from build123d import *

# Parameters (mm, degrees)
F1_DEPTH    = 6
F2_W        = 8.5644074716
F2_H        = 2.9347334579
F3_DEPTH    = 6
F5_DEPTH    = 25
F6_T1_DEPTH = 24.4869357348
F6_T3_DEPTH = 24.4827319302
F7_R        = 3
F8_R        = 1


# Not quite as in the source:
# - a fillet or chamfer that OpenCascade refuses, or shapes differently, is made with other operations: its cross-section is extruded or revolved along the edge and cut away or added


with BuildPart() as f1:
    # F0 (on Top) → F1 (new body)
    with BuildSketch(Plane.XY):
        Polygon((-4.42252215, 28.2665032521), (16.57747785, 28.2665032521), (16.57747785, -12.2334967479), (-4.42252215, -12.2334967479), (-4.42252215, -11.2334967479), (-5.42252215, -11.2334967479), (-5.42252215, -13.2334967479), (-5.42252215, -15.2334967479), (-4.42252215, -15.2334967479), (16.57747785, -15.2334967479), (19.57747785, -15.2334967479), (19.57747785, -13.2334967479), (19.57747785, 27.2665032521), (19.57747785, 31.2665032521), (16.57747785, 31.2665032521), (-4.42252215, 31.2665032521), (-5.42252215, 31.2665032521), (-5.42252215, 27.2665032521), (-4.42252215, 27.2665032521), align=None)
    extrude(amount=F1_DEPTH)

    # F2 (on face) → F3 (join)
    with BuildSketch(Plane.YZ.offset(19.57747785)):
        with Locations((7.0165032521, 3)):
            Rectangle(F2_W, F2_H)
    extrude(amount=F3_DEPTH)

    # F4 (on face) → F5 (cut)
    with BuildSketch(Plane.XY.offset(4.4673667289)):
        with BuildLine():
            Line((25.57747785, 8.833928965), (22.57747785, 9.2672181241))
            ThreePointArc((22.57747785, 9.2672181241), (20.32747785, 7.0172181241), (22.57747785, 4.7672181241))
            Line((22.57747785, 4.7672181241), (25.57747785, 5.2005072832))
            Line((25.57747785, 5.2005072832), (25.57747785, 8.833928965))
        make_face()
    extrude(amount=-F5_DEPTH, mode=Mode.SUBTRACT)

    # F6: fillet of radius 5 on 2 edges, made by hand

    # F6_s2 → F6_t1 (cut)
    with BuildSketch(Plane.XY.offset(-9.2434678674)):
        with BuildLine():
            ThreePointArc((21.2670373946, 2.7342995163), (23.7500837932, 3.3944284833), (25.57747785, 5.2005072832))
            Line((25.57747785, 5.2005072832), (25.57747785, 2.7342995163))
            Line((25.57747785, 2.7342995163), (21.2670373946, 2.7342995163))
        make_face()
    extrude(amount=F6_T1_DEPTH, mode=Mode.SUBTRACT)

    # F6_s4 → F6_t3 (cut)
    with BuildSketch(Plane.XY.offset(-9.2413659651)):
        with BuildLine():
            ThreePointArc((21.2678781556, 11.2987069879), (23.7502046967, 10.6389898062), (25.57747785, 8.833928965))
            Line((25.57747785, 8.833928965), (25.57747785, 11.2987069879))
            Line((25.57747785, 11.2987069879), (21.2678781556, 11.2987069879))
        make_face()
    extrude(amount=F6_T3_DEPTH, mode=Mode.SUBTRACT)

    # F7
    f7_edges = [f1.edges().sort_by_distance(p)[0] for p in [
        (19.577478, -15.233497, 3),
        (19.577478, 31.266503, 3),
    ]]
    fillet(f7_edges, radius=F7_R)

    # F8
    f8_edges = [f1.edges().sort_by_distance(p)[0] for p in [
        (-5.422522, -15.233497, 3),
        (-5.422522, 31.266503, 3),
        (23.750084, 3.394428, 4.467367),
        (23.750084, 3.394428, 1.532633),
        (23.750205, 10.63899, 1.532633),
        (23.750205, 10.63899, 4.467367),
        (20.422678, 11.298707, 1.532633),
        (20.422258, 2.7343, 1.532633),
        (20.422258, 2.7343, 4.467367),
        (20.422678, 11.298707, 4.467367),
    ]]
    fillet(f8_edges, radius=F8_R)


solid = f1.part
Input: part model. Units: mm. Frame: model coordinates. A direction names the side the tool comes from. Give positions to 0.01 mm unless a question says otherwise; leave off trailing zeros. Order: outer loops, then holes, each group sorted by start corner. A loop starts at its lowest first (then second) coordinate and runs counter-clockwise, first axis right, second up.
Q1. Section B-B on z = 1.05. Output: boundary loops of the cut face in (x, y), and give its area (3 significant figures).
Checked values:
outline: (-5.42, -14.23) arc R1 ccw to (-4.42, -15.23) - (16.58, -15.23) arc R3 ccw to (19.58, -12.23) - (19.58, 28.27) arc R3 ccw to (16.58, 31.27) - (-4.42, 31.27) arc R1 ccw to (-5.42, 30.27) - (-5.42, 27.27) - (-4.42, 27.27) - (-4.42, 28.27) - (16.58, 28.27) - (16.58, -12.23) - (-4.42, -12.23) - (-4.42, -11.23) - (-5.42, -11.23) - close
area: 269 mm2
Q2. Set-up query: faces 4 (the cylindrical face through (20.43, 11, 4.18)), 5 (the flat face through (20, 7, 1.533)), 6 (the flat face through (6, 28.267, 3)), 7 (the flat face through (-5, 27.267, 3)). Return all of +Z, -Z, +X, -X, +Y, -Y with unobstructed straight access to the full face (end or side cutting, diameter ignored); none if empty.
Checked values:
face 4: +Z, +X, +Y
face 5: -Z, +X, +Y, -Y
face 6: +Z, -Z
face 7: +Z, -Z, -X
Q3. Section C-C on y = 15. Output: boundary loops of the cut face in (x, z).
Checked values:
outline: (16.58, 0) - (19.58, 0) - (19.58, 6) - (16.58, 6) - close
Q4. Section A-A on x = 1. Output: boundary loops of the cut face in (y, z).
Checked values:
outline: (-15.23, 0) - (-12.23, 0) - (-12.23, 6) - (-15.23, 6) - close; (28.27, 0) - (31.27, 0) - (31.27, 6) - (28.27, 6) - close
Q5. Contact query for flat-ended pins moving along their axis: pin 1 Ø0.5 at (x, z) = (-5, 4.5) entering from +Y; pin 2 Ø0.8 at (x, z) = (-5, 4) entering from -Y; pin 3 Ø1.1 at (y, z) = (28, 4) entering from +X. Output: stop coordinate, or through.
Checked values:
pin 1: stops at y = 31.21
pin 2: stops at y = -15.22
pin 3: stops at x = 19.58
Q6. Ray query, probe 1 along Y at (x, z) = (3.5, 0.95); probe 2 along X at (y, z) = (27.5, 2.55); probe 3 along X at (y, z) = (-7, 2.9). Return the intervals inside material, ascending.
Checked values:
probe 1: y = -15.23 to -12.23, 28.27 to 31.27
probe 2: x = -5.42 to -4.42, 16.58 to 19.58
probe 3: x = 16.58 to 19.58
Q7. Draft query along Y for faces 1 (the flat face through (20, 7, 4.467)), 2 (the flat face through (20, 11.299, 3)), 3 (the cylindrical face through (20.33, 7.07, 3.02)). Return one class per face: +Y half, -Y half, draft (parallel to the pull), parting line (faces both ways), or undercut.
Checked values:
face 1: draft
face 2: +Y half
face 3: undercut
